Design review of the part built by this model. Coordinates are the model's own, in mm. A direction names the side the tool comes from. Round coordinates to 2 decimals unless told otherwise and drop trailing zeros. Order: outer loops, then holes, each group sorted by start corner. A loop starts at its lowest first (then second) coordinate and runs counter-clockwise, first axis right, second up. Notation, with made-up numbers: (84.25, 47) - (125.25, 47) arc R25 ccw to (125.25, 82) - close; hole circle Ø5 at (86.5, 47.5). An arc over 180 degrees is marked (long way). Write item = value, one per line.
from build123d import *

# Parameters (mm, degrees)
F0_W      = 211.511924
F0_H      = 121.89918
F1_DEPTH  = 41.91
F2_R      = 13.096374
F3_DEPTH  = 7.874
F4_R      = 12.492231
F5_DEPTH  = 7.874
F6_R      = 12.342141
F7_DEPTH  = 8.636
F8_R      = 12.267879
F9_DEPTH  = 7.366
F10_W     = 194.494978
F10_H     = 109.122164
F11_DEPTH = 35.56
F12_R     = 17.252828
F13_DEPTH = 40.852703
F14_R     = 16.340018
F15_DEPTH = 40.93973
F16_R     = 17.743015
F17_DEPTH = 41.344658


with BuildPart() as f1:
    # F0 (on Top) → F1 (new body)
    with BuildSketch(Plane.XY):
        Rectangle(F0_W, F0_H)
    extrude(amount=F1_DEPTH)

    # F2 (on face) → F3 (join)
    with BuildSketch(Plane.XY.offset(41.91)):
        with Locations((-78.215137, 27.114578)):
            Circle(F2_R)
    extrude(amount=F3_DEPTH)

    # F4 (on face) → F5 (join)
    with BuildSketch(Plane.XY.offset(41.91)):
        with Locations((-79.258002, -24.949349)):
            Circle(F4_R)
    extrude(amount=F5_DEPTH)

    # F6 (on face) → F7 (join)
    with BuildSketch(Plane.XY.offset(41.91)):
        with Locations((-25.289563, 27.77613)):
            Circle(F6_R)
    extrude(amount=F7_DEPTH)

    # F8 (on face) → F9 (join)
    with BuildSketch(Plane.XY.offset(41.91)):
        with Locations((-25.382636, -24.802757)):
            Circle(F8_R)
    extrude(amount=F9_DEPTH)

    # F10 (on face) → F11 (cut)
    with BuildSketch(Plane.XY):
        Rectangle(F10_W, F10_H)
    extrude(amount=F11_DEPTH, mode=Mode.SUBTRACT)

    # F12 (on face) → F13 (join)
    with BuildSketch(Plane.XY):
        Circle(F12_R)
    extrude(amount=F13_DEPTH)

    # F14 (on face) → F15 (join)
    with BuildSketch(Plane.XY):
        with Locations((-64.27452, 0)):
            Circle(F14_R)
    extrude(amount=F15_DEPTH)

    # F16 (on face) → F17 (join)
    with BuildSketch(Plane.XY):
        with Locations((55.832461, 0)):
            Circle(F16_R)
    extrude(amount=F17_DEPTH)


solid = f1.part
Item 1: The part is to be moulded in two halves that separate along X. For faces 6 (the face through (-1, 54.561, 18)), 7 (the face through (-1, -54.561, 18)), 8 (the face through (-105.756, -1, 21)), 9 (the face through (-65, 0, 0)), say which applies: +X half, -X half, draft (parallel to the pull), parting line (faces both ways), or undercut.
Data:
face_6 = undercut
face_7 = undercut
face_8 = -X half
face_9 = draft
Item 2: Take a section at C-C, the plane x = 0. State the section outline as (y, z) points.
Data:
outline = (-60.95, 0) - (-54.56, 0) - (-54.56, 35.56) - (-17.25, 35.56) - (-17.25, 0) - (17.25, 0) - (17.25, 35.56) - (54.56, 35.56) - (54.56, 0) - (60.95, 0) - (60.95, 41.91) - (-60.95, 41.91) - close
Item 3: For line 1 along Y through (x, z) = (-65.5, 25.5); line 2 along X through (y, z) = (-49, 7); line 3 along Y through (x, z) = (82.5, 11), list the stretches that pass through material, from the lowest coordinate up. Write a range as [from, to].
Data:
line_1 = [-60.95, -54.56], [-16.29, 16.29], [54.56, 60.95]
line_2 = [-105.76, -97.25], [97.25, 105.76]
line_3 = [-60.95, -54.56], [54.56, 60.95]
Item 4: For faces 1 (the face through (-91.74, -24.4, 45.79)), 2 (the face through (-25, 28, 50.546)), 3 (the face through (-26, -25, 49.276)), 4 (the face through (-49.2, -6.3, 17.5)), 5 (the face through (-78, 27, 49.784)), list the 3-axis set-ups (+Z, -Z, +X, -X, +Y, -Y) from which the entire face can be reached by the end or side of a thin tool; tool diameter is ignored.
Data:
face_1 = +Z
face_2 = +Z, +X, -X, +Y, -Y
face_3 = +Z, +X, -Y
face_4 = -Z
face_5 = +Z, -X, +Y, -Y
Item 5: Take a section at B-B, the plane y = -42.5. State the section outline as (x, z) points, and give its area (3 significant figures).
Data:
outline = (-105.76, 0) - (-97.25, 0) - (-97.25, 35.56) - (97.25, 35.56) - (97.25, 0) - (105.76, 0) - (105.76, 41.91) - (-105.76, 41.91) - close
area = 1,950 mm2
Item 6: Take a section at D-D, the plane x = 91.5. State the section outline as (y, z) points, and give its area (3 significant figures).
Data:
outline = (-60.95, 0) - (-54.56, 0) - (-54.56, 35.56) - (54.56, 35.56) - (54.56, 0) - (60.95, 0) - (60.95, 41.91) - (-60.95, 41.91) - close
area = 1,230 mm2
Item 7: Insertion check: P1, Ø12.5, axis at x = -74, y = -30, coming from the +Z side; P2, Ø1, axis at x = -56.5, y = -13.5, coming from the +Z side; P3, Ø12.5, axis at x = -28.5, y = -25.5, coming from the +Z side. Each pin has a flat end and moves straight along its axis. Give the tip position at first contact, or say it passes through.
Data:
P1 = 49.78
P2 = 41.91
P3 = 49.28
Item 8: Take a section at A-A, the plane z = 31. State the section outline as (x, y) points, and give its area (3 significant figures).
Data:
outline = (-105.76, -60.95) - (105.76, -60.95) - (105.76, 60.95) - (-105.76, 60.95) - close; circle Ø32.68 at (-64.27, 0); circle Ø34.51 at (0, 0); circle Ø35.49 at (55.83, 0); hole (-97.25, -54.56) - (97.25, -54.56) - (97.25, 54.56) - (-97.25, 54.56) - close
area = 7,320 mm2
